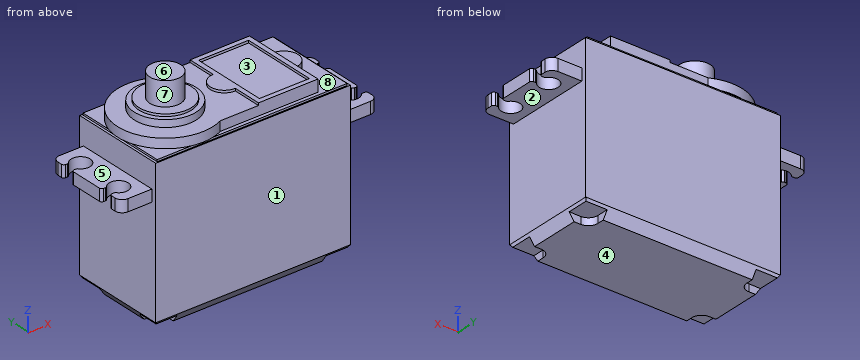
from build123d import *
from OCP.BRepFilletAPI import BRepFilletAPI_MakeChamfer

# Parameters (mm, degrees)
SKETCH1_W            = 40.9
SKETCH1_H            = 20
BOSS_EXTRUDE1_DEPTH  = 19.3
SKETCH2_W            = 40.9
SKETCH2_H            = 20
BOSS_EXTRUDE2_DEPTH  = 6.5
SKETCH3_W            = 40.9
SKETCH3_H            = 20
BOSS_EXTRUDE3_DEPTH  = 6.5
CHAMFER1_SIZE        = 2
CHAMFER1_SIZE2       = 1.400415076
CUT_EXTRUDE1_DEPTH   = 1.5
SKETCH5_W            = 39.9
SKETCH5_H            = 19.5
BOSS_EXTRUDE4_DEPTH  = 0.4
BOSS_EXTRUDE5_DEPTH  = 2
SKETCH7_R            = 6.5
BOSS_EXTRUDE6_DEPTH  = 1.5
SKETCH8_R            = 5.5
BOSS_EXTRUDE7_DEPTH  = 0.5
SKETCH9_R            = 3.25
BOSS_EXTRUDE8_DEPTH  = 5
SKETCH10_W           = 10.5
SKETCH10_H           = 15.998933302
BOSS_EXTRUDE9_DEPTH  = 0.5
BOSS_EXTRUDE10_START = -5.74
BOSS_EXTRUDE10_DEPTH = 2.5


with BuildPart() as part:
    # Sketch1 → Boss-Extrude1 (new body)
    with BuildSketch(Plane.XY):
        Rectangle(SKETCH1_W, SKETCH1_H)
    extrude(amount=BOSS_EXTRUDE1_DEPTH)

    # Sketch2 → Boss-Extrude2 (add)
    with BuildSketch(Plane(origin=(0, 0, 0), x_dir=(-1, 0, 0), z_dir=(0, 0, -1))):
        Rectangle(SKETCH2_W, SKETCH2_H)
    extrude(amount=BOSS_EXTRUDE2_DEPTH)

    # Sketch3 → Boss-Extrude3 (add)
    with BuildSketch(Plane.XY.offset(19.3)):
        Rectangle(SKETCH3_W, SKETCH3_H)
    extrude(amount=BOSS_EXTRUDE3_DEPTH)

    # Chamfer1: one chamfer whose edges measure the first distance from different faces: ONE call of the kernel's chamfer builder (chamfer() names one face for all edges)
    chamfer1_edges_1 = [part.edges().sort_by_distance(p)[0] for p in [
        (0, 10, -6.5),
    ]]
    chamfer1_side_1 = [part.faces().sort_by_distance(p)[0] for p in [
        (0, 10, 9.65),
    ]]
    chamfer1_edges_2 = [part.edges().sort_by_distance(p)[0] for p in [
        (20.45, 0, -6.5),
    ]]
    chamfer1_side_2 = [part.faces().sort_by_distance(p)[0] for p in [
        (20.45, 0, 9.65),
    ]]
    chamfer1_edges_3 = [part.edges().sort_by_distance(p)[0] for p in [
        (0, -10, -6.5),
    ]]
    chamfer1_side_3 = [part.faces().sort_by_distance(p)[0] for p in [
        (0, -10, 9.65),
    ]]
    chamfer1_edges_4 = [part.edges().sort_by_distance(p)[0] for p in [
        (-20.45, 0, -6.5),
    ]]
    chamfer1_side_4 = [part.faces().sort_by_distance(p)[0] for p in [
        (-20.45, 0, 9.65),
    ]]
    chamfer1 = BRepFilletAPI_MakeChamfer(part.part.solid().wrapped)
    for e in chamfer1_edges_1:
        chamfer1.Add(CHAMFER1_SIZE, CHAMFER1_SIZE2, e.wrapped, chamfer1_side_1[0].wrapped)  # the first distance lies on this face
    for e in chamfer1_edges_2:
        chamfer1.Add(CHAMFER1_SIZE, CHAMFER1_SIZE2, e.wrapped, chamfer1_side_2[0].wrapped)  # the first distance lies on this face
    for e in chamfer1_edges_3:
        chamfer1.Add(CHAMFER1_SIZE, CHAMFER1_SIZE2, e.wrapped, chamfer1_side_3[0].wrapped)  # the first distance lies on this face
    for e in chamfer1_edges_4:
        chamfer1.Add(CHAMFER1_SIZE, CHAMFER1_SIZE2, e.wrapped, chamfer1_side_4[0].wrapped)  # the first distance lies on this face
    add(Compound.cast(chamfer1.Shape()), mode=Mode.REPLACE)

    # Sketch4 → Cut-Extrude1 (cut)
    with BuildSketch(Plane(origin=(0, 0, -6.5), x_dir=(-1, 0, 0), z_dir=(0, 0, -1))):
        with BuildLine():
            Line((-20.45, 10), (-15.65, 10))
            Line((-15.65, 10), (-15.65, 7.2))
            ThreePointArc((-15.65, 7.2), (-16.235786438, 5.785786438), (-17.65, 5.2))
            Line((-17.65, 5.2), (-20.45, 5.2))
            Line((-20.45, 5.2), (-20.45, 10))
        make_face()
        with BuildLine():
            Line((15.65, 10), (15.65, 7.2))
            ThreePointArc((15.65, 7.2), (16.235786438, 5.785786438), (17.65, 5.2))
            Line((17.65, 5.2), (20.45, 5.2))
            Line((20.45, 5.2), (20.45, 10))
            Line((20.45, 10), (15.65, 10))
        make_face()
        with BuildLine():
            Line((20.45, -10), (15.65, -10))
            Line((15.65, -10), (15.65, -7.2))
            ThreePointArc((15.65, -7.2), (16.235786438, -5.785786438), (17.65, -5.2))
            Line((17.65, -5.2), (20.45, -5.2))
            Line((20.45, -5.2), (20.45, -10))
        make_face()
        with BuildLine():
            Line((-15.65, -10), (-15.65, -7.2))
            ThreePointArc((-15.65, -7.2), (-16.235786438, -5.785786438), (-17.65, -5.2))
            Line((-17.65, -5.2), (-20.45, -5.2))
            Line((-20.45, -5.2), (-20.45, -10))
            Line((-20.45, -10), (-15.65, -10))
        make_face()
    extrude(amount=-CUT_EXTRUDE1_DEPTH, mode=Mode.SUBTRACT)

    # Sketch5 → Boss-Extrude4 (add)
    with BuildSketch(Plane.XY.offset(25.8)):
        Rectangle(SKETCH5_W, SKETCH5_H)
    extrude(amount=BOSS_EXTRUDE4_DEPTH)

    # Sketch6 → Boss-Extrude5 (add)
    with BuildSketch(Plane.XY.offset(26.2)):
        with BuildLine():
            Line((-6.09, 8.999466651), (14.45, 8.999466651))
            Line((14.45, 8.999466651), (14.45, 3))
            ThreePointArc((14.45, 3), (17.45, 0), (14.45, -3))
            Line((14.45, -3), (14.45, -8.999466651))
            Line((14.45, -8.999466651), (-6.09, -8.999466651))
            ThreePointArc((-6.09, -8.999466651), (-20.45, 0), (-6.09, 8.999466651))
        make_face()
    extrude(amount=BOSS_EXTRUDE5_DEPTH)

    # Sketch7 → Boss-Extrude6 (add)
    with BuildSketch(Plane.XY.offset(28.2)):
        with Locations((-10.45, 0)):
            Circle(SKETCH7_R)
    extrude(amount=BOSS_EXTRUDE6_DEPTH)

    # Sketch8 → Boss-Extrude7 (add)
    with BuildSketch(Plane.XY.offset(29.7)):
        with Locations((-10.45, 0)):
            Circle(SKETCH8_R)
    extrude(amount=BOSS_EXTRUDE7_DEPTH)

    # Sketch9 → Boss-Extrude8 (add)
    with BuildSketch(Plane.XY.offset(30.2)):
        with Locations((-10.45, 0)):
            Circle(SKETCH9_R)
    extrude(amount=BOSS_EXTRUDE8_DEPTH)

    # Sketch10 → Boss-Extrude9 (add)
    with BuildSketch(Plane.XY.offset(28.2)):
        with BuildLine():
            Line((1.95, 8.999466651), (14.45, 8.999466651))
            Line((14.45, 8.999466651), (14.45, -8.999466651))
            Line((14.45, -8.999466651), (1.95, -8.999466651))
            Line((1.95, -8.999466651), (1.95, -2.925))
            ThreePointArc((1.95, -2.925), (-0.975, 0), (1.95, 2.925))
            Line((1.95, 2.925), (1.95, 8.999466651))
        make_face()
        with Locations((8.2, 0)):
            Rectangle(SKETCH10_W, SKETCH10_H, mode=Mode.SUBTRACT)
    extrude(amount=BOSS_EXTRUDE9_DEPTH)

    # Sketch11 → Boss-Extrude10 (add)
    with BuildSketch(Plane.XY.offset(26.2).offset(BOSS_EXTRUDE10_START)):
        with BuildLine():
            Line((20.45, 9), (25.5, 9))
            ThreePointArc((25.5, 9), (26.560660172, 8.560660172), (27, 7.5))
            Line((27, 7.5), (27, 6.601517979))
            ThreePointArc((27, 6.601517979), (26.853553391, 6.247964588), (26.5, 6.101517979))
            Line((26.5, 6.101517979), (26.150343239, 6.101517979))
            ThreePointArc((26.150343239, 6.101517979), (25.938390176, 6.148664914), (25.766408861, 6.281214383))
            ThreePointArc((25.766408861, 6.281214383), (22.23067135, 5), (25.766408861, 3.718785617))
            ThreePointArc((25.766408861, 3.718785617), (25.938390176, 3.851335086), (26.150343239, 3.898482021))
            Line((26.150343239, 3.898482021), (26.5, 3.898482021))
            ThreePointArc((26.5, 3.898482021), (26.853553391, 3.752035412), (27, 3.398482021))
            Line((27, 3.398482021), (27, -3.398482021))
            ThreePointArc((27, -3.398482021), (26.853553391, -3.752035412), (26.5, -3.898482021))
            Line((26.5, -3.898482021), (26.150343239, -3.898482021))
            ThreePointArc((26.150343239, -3.898482021), (25.938390176, -3.851335086), (25.766408861, -3.718785617))
            ThreePointArc((25.766408861, -3.718785617), (22.23067135, -5), (25.766408861, -6.281214383))
            ThreePointArc((25.766408861, -6.281214383), (25.938390176, -6.148664914), (26.150343239, -6.101517979))
            Line((26.150343239, -6.101517979), (26.5, -6.101517979))
            ThreePointArc((26.5, -6.101517979), (26.853553391, -6.247964588), (27, -6.601517979))
            Line((27, -6.601517979), (27, -7.5))
            ThreePointArc((27, -7.5), (26.560660172, -8.560660172), (25.5, -9))
            Line((25.5, -9), (20.45, -9))
            Line((20.45, -9), (20.45, 9))
        make_face()
        with BuildLine():
            Line((-20.45, -9), (-25.5, -9))
            ThreePointArc((-25.5, -9), (-26.560660172, -8.560660172), (-27, -7.5))
            Line((-27, -7.5), (-27, -6.601517979))
            ThreePointArc((-27, -6.601517979), (-26.853553391, -6.247964588), (-26.5, -6.101517979))
            Line((-26.5, -6.101517979), (-26.150343239, -6.101517979))
            ThreePointArc((-26.150343239, -6.101517979), (-25.938390176, -6.148664914), (-25.766408861, -6.281214383))
            ThreePointArc((-25.766408861, -6.281214383), (-22.23067135, -5), (-25.766408861, -3.718785617))
            ThreePointArc((-25.766408861, -3.718785617), (-25.938390176, -3.851335086), (-26.150343239, -3.898482021))
            Line((-26.150343239, -3.898482021), (-26.5, -3.898482021))
            ThreePointArc((-26.5, -3.898482021), (-26.853553391, -3.752035412), (-27, -3.398482021))
            Line((-27, -3.398482021), (-27, 3.398482021))
            ThreePointArc((-27, 3.398482021), (-26.853553391, 3.752035412), (-26.5, 3.898482021))
            Line((-26.5, 3.898482021), (-26.150343239, 3.898482021))
            ThreePointArc((-26.150343239, 3.898482021), (-25.938390176, 3.851335086), (-25.766408861, 3.718785617))
            ThreePointArc((-25.766408861, 3.718785617), (-22.23067135, 5), (-25.766408861, 6.281214383))
            ThreePointArc((-25.766408861, 6.281214383), (-25.938390176, 6.148664914), (-26.150343239, 6.101517979))
            Line((-26.150343239, 6.101517979), (-26.5, 6.101517979))
            ThreePointArc((-26.5, 6.101517979), (-26.853553391, 6.247964588), (-27, 6.601517979))
            Line((-27, 6.601517979), (-27, 7.5))
            ThreePointArc((-27, 7.5), (-26.560660172, 8.560660172), (-25.5, 9))
            Line((-25.5, 9), (-20.45, 9))
            Line((-20.45, 9), (-20.45, -9))
        make_face()
    extrude(amount=-BOSS_EXTRUDE10_DEPTH)


solid = part.part
The listing builds one solid part. Answer for the finished solid, in the listing's coordinates (mm). Face numbers are marked on the shaded views. A direction names the side the tool comes from. Round coordinates to 2 decimals unless told otherwise and drop trailing zeros. Write each loop counter-clockwise with the first axis right and the second up, starting at its lowest first coordinate (ties: lowest second). Pieces come first, ordered by that corner, then holes. Notation, with made-up numbers: M 37,10 L 75,10 A20 cw 75,25 Z; hole C 2,37 d5. An arc over 180 degrees is marked long. Write each question's results on one line, items separated by ' | '. Start each with the question number.
Item 1: The mould has two halves that part along Y. Classify the marked faces 1, 2 and 3: +Y half, -Y half, draft (parallel to the pull), parting line (faces both ways), or undercut.
Item 2: Find section B-B on z = 11. Write down the section's boundary in (x, y).
Item 3: Given pin 1 Ø4 at (y, z) = (-3.5, 8) entering from +X; pin 2 Ø3.5 at (x, y) = (23, 3.5) entering from +Z; pin 3 Ø1.2 at (y, z) = (-8, -5.5) entering from -X, each flat-ended and moving along its own axis, determine where each tip first touches the part or whether it passes through.
Item 4: Straight lines are drawn through the part: probe 1 along X at (y, z) = (-6.25, 3); probe 2 along Z at (x, y) = (-7, -8); probe 3 along Z at (x, y) = (16, -3). For each, find the intervals that lie inside material, in ascending order.
Item 5: Find section A-A on x = -10.45. Write down the section's boundary in (y, z), and give its area (4 significant figures).
Item 6: Which of the six approach directions +Z, -Z, +X, -X, +Y, -Y give full straight-line access (tool end or side, diameter ignored) to the marked faces 4, 5, 6, 7 and 8?
Answer block:
1) face 1: -Y half | face 2: draft | face 3: undercut
2) outline: M -20.45,-10 L 20.45,-10 L 20.45,10 L -20.45,10 Z
3) pin 1: stops at x = 20.45 | pin 2: stops at z = 20.46 | pin 3: stops at x = -20.17
4) probe 1: x = -20.45 to 20.45 | probe 2: z = -6.5 to 28.2 | probe 3: z = -6.5 to 26.2
5) outline: M -10,-4.5 L -8.6,-6.5 L 8.6,-6.5 L 10,-4.5 L 10,25.8 L 9.75,25.8 L 9.75,26.2 L 10,26.2 L 10,28.2 L 6.5,28.2 L 6.5,29.7 L 5.5,29.7 L 5.5,30.2 L 3.25,30.2 L 3.25,35.2 L -3.25,35.2 L -3.25,30.2 L -5.5,30.2 L -5.5,29.7 L -6.5,29.7 L -6.5,28.2 L -10,28.2 L -10,26.2 L -9.75,26.2 L -9.75,25.8 L -10,25.8 Z | area: 748.5 mm²
6) face 4: -Z, +X, -X, +Y, -Y | face 5: +Z, -X, +Y, -Y | face 6: +Z, +X, -X, +Y, -Y | face 7: +Z | face 8: +Z, +X
